```python
from build123d import *

# Parameters (mm, degrees)
SKETCH_1_W                  = 155
SKETCH_1_H                  = 45
EXTRUDE_1_DEPTH             = 5
SKETCH_2_W                  = 144
SKETCH_2_H                  = 34
CUT_EXTRUDE_1_DEPTH         = 3
FILLET_1_R                  = 5
FILLET_2_R                  = 5
SKETCH_7_W                  = 22.5
SKETCH_7_H                  = 5.5
CUT_EXTRUDE_2_DEPTH         = 3
FILLET_7_R                  = 1.2
SKETCH_9_W                  = 12
SKETCH_9_H                  = 5.5
CUT_EXTRUDE_3_DEPTH         = 3
HOLE_WIZARD_2_1_2_1_2_D     = 2.1
HOLE_WIZARD_2_1_2_1_2_DEPTH = 13.2
HOLE_WIZARD_2_1_2_1_2_TIP   = 0.63090365
SKETCH_15_W                 = 12
SKETCH_15_H                 = 5.5
CUT_EXTRUDE_4_DEPTH         = 3


with BuildPart() as part:
    # 草图1 → 凸台-拉伸1 (new body)
    with BuildSketch(Plane.XY):
        Rectangle(SKETCH_1_W, SKETCH_1_H)
    extrude(amount=EXTRUDE_1_DEPTH)

    # 草图2 → 切除-拉伸1 (cut)
    with BuildSketch(Plane.XY.offset(5)):
        Rectangle(SKETCH_2_W, SKETCH_2_H)
    extrude(amount=-CUT_EXTRUDE_1_DEPTH, mode=Mode.SUBTRACT)

    # 圆角1
    fillet_1_edges = [part.edges().sort_by_distance(p)[0] for p in [
        (-77.5, 22.5, 2.5),
        (77.5, 22.5, 2.5),
    ]]
    fillet(fillet_1_edges, radius=FILLET_1_R)

    # 圆角2
    fillet_2_edges = [part.edges().sort_by_distance(p)[0] for p in [
        (-72, -17, 3.5),
        (-72, 17, 3.5),
        (72, 17, 3.5),
        (72, -17, 3.5),
    ]]
    fillet(fillet_2_edges, radius=FILLET_2_R)

    # 草图7 → 切除-拉伸2 (cut)
    with BuildSketch(Plane.XY.offset(5)):
        with Locations((-6.895727583, -19.75)):
            Rectangle(SKETCH_7_W, SKETCH_7_H)
    extrude(amount=-CUT_EXTRUDE_2_DEPTH, mode=Mode.SUBTRACT)

    # 圆角7
    fillet_7_edges = [part.edges().sort_by_distance(p)[0] for p in [
        (-6.895727583, -22.5, 2),
    ]]
    fillet(fillet_7_edges, radius=FILLET_7_R)

    # 草图9 → 切除-拉伸3 (cut)
    with BuildSketch(Plane.XY.offset(5)):
        with Locations((16.354272417, -19.75)):
            Rectangle(SKETCH_9_W, SKETCH_9_H)
    extrude(amount=-CUT_EXTRUDE_3_DEPTH, mode=Mode.SUBTRACT)

    # 草图11 → Ø2.1 (2.1) 直径孔1 (revolve, cut)
    with BuildSketch(Plane(origin=(10.354272417, -19.75, 3.5), x_dir=(0, 0, -1), z_dir=(0, 1, 0))):
        Polygon((0, 0), (0, 36.63090365), (1.05, 36), (1.05, 0), align=None)
    revolve(axis=Axis((16.704272417, -19.75, 3.5), (-1, 0, 0)), mode=Mode.SUBTRACT)

    # Ø2.1 (2.1) 直径孔2
    with Locations(Plane(origin=(0, 22.5, 0), x_dir=(1, 0, 0), z_dir=(0, 1, 0))):
        with Locations((0, -3.5), (-7.5, -3.5)):
            Hole(HOLE_WIZARD_2_1_2_1_2_D / 2, depth=HOLE_WIZARD_2_1_2_1_2_DEPTH)
            with Locations((0, 0, -(HOLE_WIZARD_2_1_2_1_2_DEPTH + HOLE_WIZARD_2_1_2_1_2_TIP / 2))):  # 118° drill point
                Cone(0, HOLE_WIZARD_2_1_2_1_2_D / 2, HOLE_WIZARD_2_1_2_1_2_TIP, mode=Mode.SUBTRACT)

    # 草图15 → 切除-拉伸4 (cut)
    with BuildSketch(Plane.XY.offset(5)):
        with Locations((-30.145727583, -19.75)):
            Rectangle(SKETCH_15_W, SKETCH_15_H)
    extrude(amount=-CUT_EXTRUDE_4_DEPTH, mode=Mode.SUBTRACT)


solid = part.part
```
Geometry: final body of the model. Coordinates: model frame, mm. A direction names the side the tool comes from. Coordinates: 2 decimals unless noted, no trailing zeros. Order: outer loops, then holes, each group sorted by start corner. A loop starts at its lowest first (then second) coordinate and runs counter-clockwise, first axis right, second up. Notation, with made-up numbers: (-10.75, 4) - (40.25, 4) arc R22 ccw to (40.25, 10) - close; hole circle Ø2 at (45, 32). An arc over 180 degrees is marked (long way). Write each question's results on one line, items separated by ' | '.
(1) First-contact query: pin 1 Ø8 at (x, y) = (46.5, -2) entering from +Z; pin 2 Ø1.3 at (x, z) = (0, 3.5) entering from +Y. Flat tips, straight axial feed; report the tip coordinate or a pass-through.
Values found:
pin 1: stops at z = 2 | pin 2: passes through
(2) Mould query, pull axis X, two halves, no side actions, for faces 1 (the face through (-24.146, -20.4, 4.52)), 2 (the face through (-77.5, -3, 2)), 3 (the face through (7, -20, 5)). Classes: +X half, -X half, draft (parallel to the pull), parting line (faces both ways), or undercut.
Values found:
face 1: undercut | face 2: -X half | face 3: draft
(3) Set-up query: faces 4 (the face through (0, 18, 5)), 5 (the face through (7, -17, 4)), 6 (the face through (10.354, -20.4, 4.52)). Return all of +Z, -Z, +X, -X, +Y, -Y with unobstructed straight access to the full face (end or side cutting, diameter ignored); none if empty.
Values found:
face 4: +Z, +X, -X, +Y, -Y | face 5: +Z | face 6: +Z, -Y
(4) Line query: line 1 (X direction, y = -18.5, z = 3.4); line 2 (Y direction, x = 8.5, z = 3.5); line 3 (Z direction, x = 0, y = 19.3). Output: solid intervals per line, ascending. Write a range as [from, to].
Values found:
line 1: x = [-77.5, -36.15], [-24.15, -18.15], [4.35, 10.35], [22.35, 77.5] | line 2: y = [-22.5, -20.8], [-18.7, -17], [17, 22.5] | line 3: z = [0, 2.45], [4.55, 5]
(5) Section query B-B, the plane z = 3.5. Count the separate pieces of the cut face and the enclosed holes in it, plus the area to 3 significant figures.
Values found:
separate pieces: 7 | enclosed holes: 0 | area: 1,790 mm²
(6) Section query A-A, the plane y = 2. Return the cut outline in (x, z), plus the area to 3 significant figures.
Values found:
outline: (-77.5, 0) - (77.5, 0) - (77.5, 5) - (72, 5) - (72, 2) - (-72, 2) - (-72, 5) - (-77.5, 5) - close | area: 343 mm²
